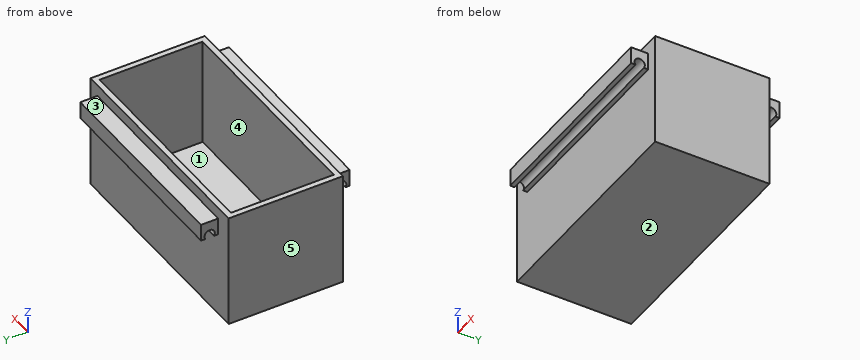
Autodesk Fusion 360 part; units mm, degrees
sketch "Esquisse1" plane through (0, 0, 0) normal (0, 0, 1) x (1, 0, 0)
  line L0 (-20, 20) -> (180, 20)
  line L1 (180, 20) -> (180, -80)
  line L2 (180, -80) -> (-20, -80)
  line L3 (-20, -80) -> (-20, 20)
  dimension "d7" = 200
  dimension "d8" = 100
sketch "Esquisse2" plane through (180, 0, 0) normal (1, 0, 0) x (0, 1, 0)
  line L0 (-80, 0) -> (20, 0)
  line L1 (20, 0) -> (20, 100)
  line L2 (20, 100) -> (-80, 100)
  line L3 (-80, 100) -> (-80, 0)
  circle A0 centre (-105, 61.7948) radius 25
  dimension "d13" = 50
sketch "Esquisse3" plane through (0, 0, 0) normal (0, 0, 1) x (1, 0, 0)
  line L0 (100, 50) -> (-100, 50)
  line L1 (-100, 50) -> (-100, -50)
  line L2 (-100, -50) -> (100, -50)
  line L3 (100, -50) -> (100, 50)
  line L4 (100, 50) -> (-100, -50) construction
  line L5 (-100, 50) -> (100, -50) construction
  dimension "d16" = 200
  dimension "d17" = 100
extrude "Extrusion3" add sketch "Esquisse3" along normal blind 100
shell "Coque2" thickness 5 removed faces 1 at (-33.3333, 16.6667, 100)
sketch "Esquisse4" plane through (0, -50, 0) normal (0, -1, 0) x (1, 0, 0)
  line L0 (-100, 0) -> (100, 0)
  line L1 (100, 0) -> (100, 100)
  line L2 (100, 100) -> (-100, 100)
  line L3 (-100, 100) -> (-100, 0)
  line L4 (-85, 90) -> (90, 90)
  line L5 (90, 90) -> (90, 75)
  line L6 (90, 75) -> (-85, 75)
  line L7 (-85, 90) -> (-85, 75)
extrude "Extrusion4" add sketch "Esquisse4" along normal blind 15 contours L4 L5 L6 L7
sketch "Esquisse5" plane through (90, 0, 0) normal (1, 0, 0) x (0, 1, 0)
  line L0 (-50, 75) -> (-50, 90)
  line L1 (-50, 90) -> (-65, 90)
  line L2 (-65, 90) -> (-65, 75)
  line L3 (-65, 75) -> (-50, 75)
  circle A0 centre (-57.5, 77.5132) radius 4.5
  dimension "d23" = 9
extrude "Extrusion5" cut sketch "Esquisse5" against normal blind 180 contours L3 A0 picked at (-57.7191, 77.5283)
mirror "Symétrie miroir1" about plane through (0, 0, 0) normal (0, 1, 0) of "Extrusion4", "Extrusion5"
extrude "Extrusion2" [suppressed]
equation "largeur = 100 mm"
equation "hauteur = 100 mm"
equation "longueur = 200 mm"
equation "epaisseurb = 5 mm"
equation "rayon = 50 mm"
equation "fixation = 5 mm"
equation "d7 = longueur"
equation "d8 = largeur"
equation "epaisseurinterieur = 5 mm"
equation "d13 = rayon"
equation "d16 = longueur"
equation "d17 = largeur"
equation "d18 = hauteur"
equation "d20 = epaisseurinterieur"
Geometry check sheet. Reference: the model listing, model coordinates, mm. Face numbers are marked on the shaded views. A direction names the side the tool comes from. Give positions to 0.01 mm unless a question says otherwise; leave off trailing zeros. Loops run counter-clockwise (first coordinate to the right, second up) from the corner with the lowest first, then second, coordinate; pieces in that order, holes last. Notation, with made-up numbers: M 76,88 L 90,88 A22 cw 90,126 Z; hole C 19,19 d9. An arc over 180 degrees is marked long. Write each question's results on one line, items separated by ' | '.
1) Section check D-D, the plane y = 21. Record the boundary of the cut face in (x, z).
Answers follow:
outline: M -100,0 L 100,0 L 100,100 L 95,100 L 95,5 L -95,5 L -95,100 L -100,100 Z
2) Section check A-A, the plane z = 79.5. Record the boundary of the cut face in (x, y).
Answers follow:
outline: M -100,-50 L -85,-50 L -85,-53.46 L 90,-53.46 L 90,-50 L 100,-50 L 100,50 L 90,50 L 90,53.46 L -85,53.46 L -85,50 L -100,50 Z; M -85,-65 L 90,-65 L 90,-61.54 L -85,-61.54 Z; M -85,61.54 L 90,61.54 L 90,65 L -85,65 Z; hole M -95,-45 L 95,-45 L 95,45 L -95,45 Z
3) Thickness scan on line 1 (Y direction, x = -41, z = 84); line 2 (X direction, y = -2, z = 24.5); line 3 (Y direction, x = 38.5, z = 78.5). Record the ranges inside material, lowest first.
Answers follow:
line 1: -65 to -45, 45 to 65 | line 2: -100 to -95, 95 to 100 | line 3: -65 to -61.89, -53.11 to -45, 45 to 53.11, 61.89 to 65
4) Tool access check on the marked faces 1 and 2. Record the directions out of +Z, -Z, +X, -X, +Y, -Y that give a thin tool (end or side, any length) a straight path to the whole face; none if there is none.
Answers follow:
face 1: +Z | face 2: -Z, +X, -X, +Y, -Y
5) Section check B-B, the plane z = 18. Record the boundary of the cut face in (x, y), plus the area to 3 significant figures.
Answers follow:
outline: M -100,-50 L 100,-50 L 100,50 L -100,50 Z; hole M -95,-45 L 95,-45 L 95,45 L -95,45 Z | area: 2,900 mm2
6) Release check for a two-part mould opening along X. For the marked faces 3, 4 and 5 record: +X half, -X half, draft (parallel to the pull), parting line (faces both ways), or undercut.
Answers follow:
face 3: draft | face 4: undercut | face 5: -X half
7) Section check C-C, the plane x = -63. Record the boundary of the cut face in (y, z).
Answers follow:
outline: M -65,75 L -61.23,75 A4.5 cw long -53.77,75 L -50,75 L -50,0 L 50,0 L 50,75 L 53.77,75 A4.5 cw long 61.23,75 L 65,75 L 65,90 L 50,90 L 50,100 L 45,100 L 45,5 L -45,5 L -45,100 L -50,100 L -50,90 L -65,90 Z
8) Gauge pin test, flat ends, axial feed: pin 1 (7.5 mm diameter, centred on x = 38.5, y = -56, fed in from +Z); pin 2 (4.5 mm diameter, centred on y = -61, z = 85.5, fed in from -X); pin 3 (1.9 mm diameter, centred on x = 20, y = -52.5, fed in from -Z); pin 4 (12 mm diameter, centred on x = 71, y = -27.5, fed in from -Z). Record the tip position at first contact, or that the pin passes through.
Answers follow:
pin 1: z = 90 | pin 2: x = -85 | pin 3: z = 75 | pin 4: z = 0
